Design review of the part built by this model. Coordinates are the model's own, in mm. Face numbers are marked on the shaded views. A direction names the side the tool comes from. Give positions to 0.01 mm unless a question says otherwise; leave off trailing zeros. Write each loop counter-clockwise with the first axis right and the second up, starting at its lowest first coordinate (ties: lowest second). Pieces come first, ordered by that corner, then holes. Notation, with made-up numbers: M 70,42 L 125,42 A23 ccw 125,60 Z; hole C -7,86 d7. An arc over 180 degrees is marked long. Answer in a Markdown table with one row per item.
```python
from build123d import *

# Parameters (mm, degrees)
MEMBER_8509_86_125_125_8_1_DEPTH = 100


with BuildPart() as part:
    # Sketch11 → Member 8509-86 125_125_8_1 (new body)
    with BuildSketch(Plane.YZ):
        with BuildLine():
            Line((-33.6, -33.6), (-33.6, 91.4))
            Line((-33.6, 91.4), (-30.2, 91.4))
            ThreePointArc((-30.2, 91.4), (-26.947308807, 90.052691193), (-25.6, 86.8))
            Line((-25.6, 86.8), (-25.6, -11.6))
            ThreePointArc((-25.6, -11.6), (-21.499494937, -21.499494937), (-11.6, -25.6))
            Line((-11.6, -25.6), (86.8, -25.6))
            ThreePointArc((86.8, -25.6), (90.052691193, -26.947308807), (91.4, -30.2))
            Line((91.4, -30.2), (91.4, -33.6))
            Line((91.4, -33.6), (-33.6, -33.6))
        make_face()
    extrude(amount=MEMBER_8509_86_125_125_8_1_DEPTH)


solid = part.part
```
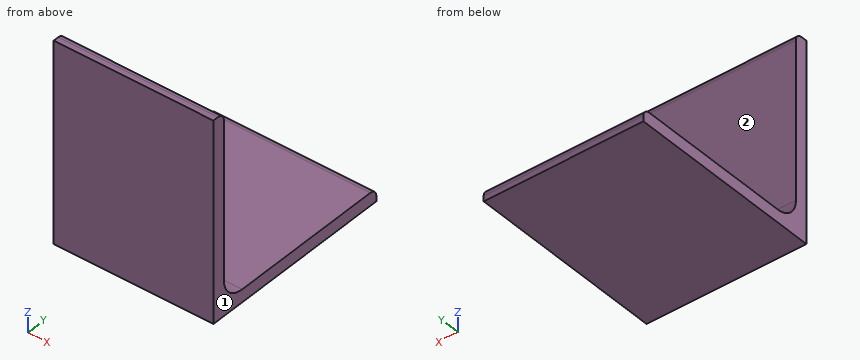
1) To check wall thickness, follow probe 1 along Y at (x, z) = (95.5, 44); probe 2 along Y at (x, z) = (83.5, -18.5). State the ranges of each line that lie inside material, in increasing order. Write a range as [from, to].
Geometry says:
| item | result |
|---|---|
| probe 1 | [-33.6, -25.6] |
| probe 2 | [-33.6, -23.78] |
2) Insertion check: P1, Ø5, axis at x = 16.5, y = 45, coming from the +Z side; P2, Ø10, axis at x = 56.5, z = 45, coming from the +Y side. Each pin has a flat end and moves straight along its axis. Give the tip position at first contact, or say it passes through.
Geometry says:
| item | result |
|---|---|
| P1 | z = -25.6 |
| P2 | y = -25.6 |
3) For the marked faces 1 and 2, list the 3-axis set-ups (+Z, -Z, +X, -X, +Y, -Y) from which the entire face can be reached by the end or side of a thin tool; tool diameter is ignored.
Geometry says:
| item | result |
|---|---|
| face 1 | +Z, -Z, +X, +Y, -Y |
| face 2 | +Z, +X, -X, +Y |
4) Add section A-A (x = 21). Write out the cut boundary in (y, z).
Geometry says:
| item | result |
|---|---|
| outline | M -33.6,-33.6 L 91.4,-33.6 L 91.4,-30.2 A4.6 ccw 86.8,-25.6 L -11.6,-25.6 A14 cw -25.6,-11.6 L -25.6,86.8 A4.6 ccw -30.2,91.4 L -33.6,91.4 Z |
5) Add section B-B (y = 54). Write out the cut boundary in (x, z), and give its area (3 significant figures).
Geometry says:
| item | result |
|---|---|
| outline | M 0,-33.6 L 100,-33.6 L 100,-25.6 L 0,-25.6 Z |
| area | 800 mm^2 |
